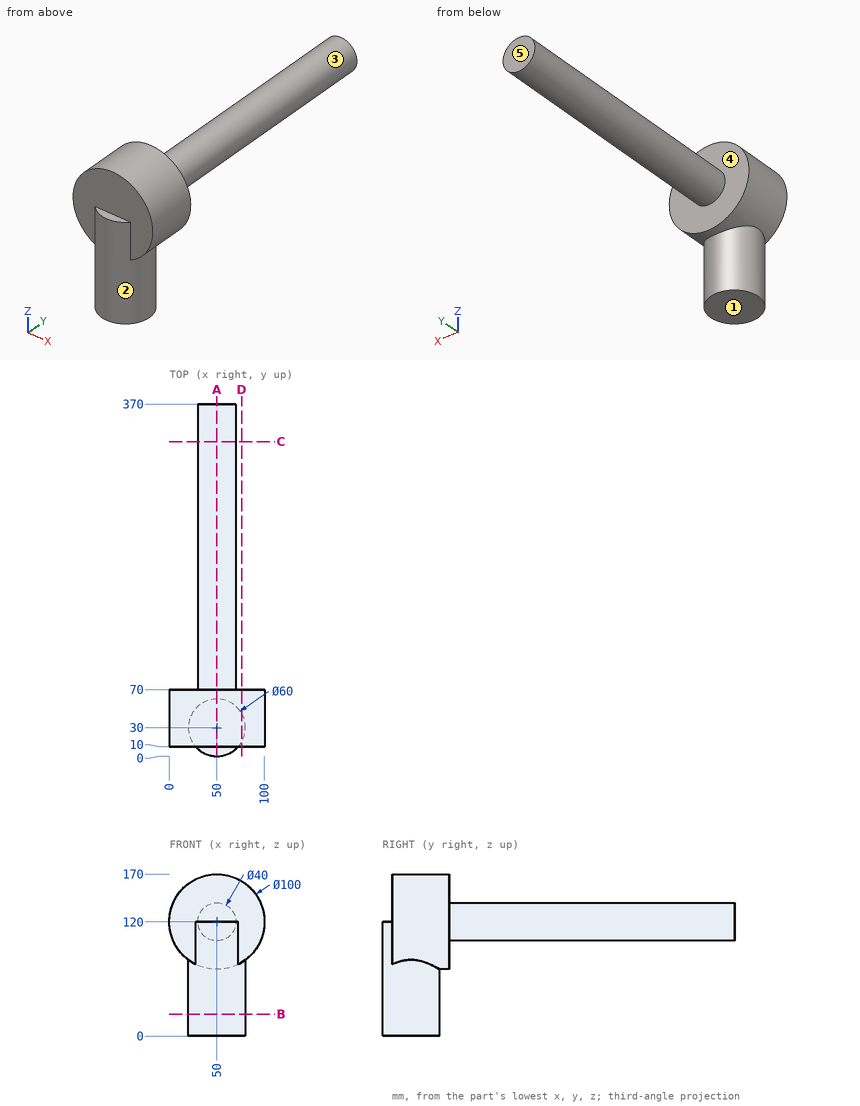
Could you check a few things on this drawing? It's one solid part, dimensions in mm from its lowest x, y, z. A direction names the side the tool comes from. Coordinates: 2 decimals unless noted, no trailing zeros. Order: outer loops, then holes, each group sorted by start corner. A loop starts at its lowest first (then second) coordinate and runs counter-clockwise, first axis right, second up. Notation, with made-up numbers: M -18,33.5 L 40,33.5 A22 ccw 40,47.5 Z; hole C -11,-28 d11. An arc over 180 degrees is marked long. Answer as a JSON object with one key per item and string values. Group by question number.
(1) Suppose I cut it at D-D, the plane x = 76. Please give me the cut outline in (y, z).
(2) For pin 1 (3 mm diameter, centred on x = 60, y = 194.5, fed in from -Z); pin 2 (4 mm diameter, centred on x = 64.5, z = 91, fed in from +Y); pin 3 (5 mm diameter, centred on x = 68.5, y = 124.5, fed in from +Z), each with a flat end and sliding along its axis, tell me the tip position at first contact or that it passes through.
(3) I need wall thicknesses on probe 1 along Y at (x, z) = (16, 121.5); probe 2 along X at (y, z) = (21, 121.5); probe 3 along X at (y, z) = (29, 28). Which ranges of each line are inside material? Lowest first, please.
(4) Which directions (+Z, -Z, +X, -X, +Y, -Y) give clear straight access to the entire face, cutting with the end or side of a thin tool? Please do the marked faces 4 and 5.
(5) Suppose I cut it at B-B, the plane z = 23. Please give me the cut outline in (x, y), then the cut area to 3 significant figures.
(6) If we mould it in two halves opening along Z, with no side actions, what happens to the marked faces 1, 2 and 3? For each: released by +Z, released by -Z, zero draft, split by the parting line, or undercut.
(7) Suppose I cut it at A-A, the plane x = 50. Please give me the cut outline in (y, z).
(8) Suppose I cut it at C-C, the plane y = 330.5. Please give me the cut outline in (x, z), then the cut area to 3 significant figures.
Values found:
{
 "1": {"outline": "M 10,77.29 L 15.03,77.29 L 15.03,0 L 44.97,0 L 44.97,77.29 L 70,77.29 L 70,162.71 L 10,162.71 Z"},
 "2": {"pin 1": "stops at z = 101.9", "pin 2": "stops at y = 70", "pin 3": "stops at z = 132"},
 "3": {"probe 1": "y = 10 to 70", "probe 2": "x = 0.02 to 99.98", "probe 3": "x = 20.02 to 79.98"},
 "4": {"face 4": "+Y", "face 5": "+Z, -Z, +X, -X, +Y"},
 "5": {"outline": "C 50,30 d60", "area": "2,830 mm^2"},
 "6": {"face 1": "released by -Z", "face 2": "zero draft", "face 3": "split by the parting line"},
 "7": {"outline": "M 0,0 L 60,0 L 60,70 L 70,70 L 70,100 L 370,100 L 370,140 L 70,140 L 70,170 L 10,170 L 10,120 L 0,120 Z"},
 "8": {"outline": "C 50,120 d40", "area": "1,260 mm^2"}
}
